```python
from build123d import *

# Parameters (mm, degrees)
SKETCH1_R           = 14.3
SKETCH1_R_2         = 12.7
BOSS_EXTRUDE1_DEPTH = 3.175
BOSS_EXTRUDE2_START = -0.635
SKETCH2_R           = 1.5875
BOSS_EXTRUDE2_DEPTH = 6.35
CIRPATTERN1_COUNT   = 2


with BuildPart() as part:
    # Sketch1 → Boss-Extrude1 (new body)
    with BuildSketch(Plane.XY):
        Circle(SKETCH1_R)
        Circle(SKETCH1_R_2, mode=Mode.SUBTRACT)
    extrude(amount=BOSS_EXTRUDE1_DEPTH)

    # Sketch2 → Boss-Extrude2 (add)
    with BuildSketch(Plane(origin=(14.3, 0, 0), x_dir=(0, 0, -1), z_dir=(1, 0, 0)).offset(BOSS_EXTRUDE2_START)):
        with Locations((-1.5875, 0)):
            Circle(SKETCH2_R)
    boss_extrude2 = extrude(amount=BOSS_EXTRUDE2_DEPTH)

    # CirPattern1: Boss-Extrude2 ×2 about axis
    cirpattern1_axis = Axis((0, 0, 3.175), (0, 0, -1))
    for i in range(1, CIRPATTERN1_COUNT):
        add(boss_extrude2.rotate(cirpattern1_axis, i * 360 / CIRPATTERN1_COUNT))


solid = part.part
```
Read the model definition and answer for the solid it produces. Units are mm, in the model's axes. A direction names the side the tool comes from. Give positions to 0.01 mm unless a question says otherwise; leave off trailing zeros. Write each loop counter-clockwise with the first axis right and the second up, starting at its lowest first coordinate (ties: lowest second). Pieces come first, ordered by that corner, then holes. Notation, with made-up numbers: (-36, -23.75) -> (10, -23.75) arc R10 ccw to (10, -13.75) -> close; hole circle Ø8 at (-11, -7). An arc over 180 degrees is marked (long way). Answer as a JSON object with one key per item and string values.
1) Straight lines are drawn through the part: probe 1 along Y at (x, z) = (0, 2.15); probe 2 along X at (y, z) = (-10, 2.05); probe 3 along X at (y, z) = (0.25, 0.35) (3 decimals). For each, find the intervals that lie inside material, in ascending order. Write a range as from..to.
Findings below:
{"probe 1": "y = -14.3..-12.7, 12.7..14.3", "probe 2": "x = -10.22..-7.83, 7.83..10.22", "probe 3": "x = -20.015..-12.698, 12.698..20.015"}
2) Section A-A on x = 0 is taken. Write down the section's boundary in (y, z) (3 decimals), then the cut area to 3 significant figures.
Findings below:
{"outline": "(-14.3, 0) -> (-12.7, 0) -> (-12.7, 3.175) -> (-14.3, 3.175) -> close; (12.7, 0) -> (14.3, 0) -> (14.3, 3.175) -> (12.7, 3.175) -> close", "area": "10.2 mm^2"}
3) For a pull along Y with two mould halves and no side action, classify faces 3 (the cylindrical face through (-2.75, -12.4, 1.57)), 4 (the cylindrical face through (-17.07, 0.61, 0.12)), 5 (the flat face through (20.015, 0, 2)) as pulls with the +Y half, pulls with the -Y half, needs draft (parallel to the pull), parting line crosses it, or undercut.
Findings below:
{"face 3": "undercut", "face 4": "parting line crosses it", "face 5": "needs draft"}
4) Flat-ended cylindrical pins translate along their axes: pin 1 Ø1 at (y, z) = (9.5, 1) entering from -X; pin 2 Ø1.5 at (x, z) = (-5.5, 1) entering from +Y; pin 3 Ø1.5 at (x, z) = (-1.5, 2.5) entering from -Y. Find the tip coordinate at first contact, or state that the pin passes through.
Findings below:
{"pin 1": "stops at x = -11.11", "pin 2": "stops at y = 13.49", "pin 3": "stops at y = -14.28"}
5) A tool of negligible diameter and unlimited length cuts with its end or side. For faces 1 (the cylindrical face through (17, 0, 0)), 2 (the flat face through (0, 13, 3.175)), from which of +Z, -Z, +X, -X, +Y, -Y can it reach the whole face along a straight path? Write none if from no direction.
Findings below:
{"face 1": "+X", "face 2": "+Z, +X, -X, +Y, -Y"}
6) Section C-C on y = 11.5 is taken. Write down the section's boundary in (x, z) (3 decimals), then the cut area to 3 significant figures.
Findings below:
{"outline": "(-8.499, 0) -> (-5.389, 0) -> (-5.389, 3.175) -> (-8.499, 3.175) -> close; (5.389, 0) -> (8.499, 0) -> (8.499, 3.175) -> (5.389, 3.175) -> close", "area": "19.8 mm^2"}
7) Section B-B on z = 1.5 is taken. Write down the section's boundary in (x, y) (3 decimals), then the cut area to 3 significant figures.
Findings below:
{"outline": "(-20.015, -1.585) -> (-14.212, -1.585) arc R14.3 ccw to (14.212, -1.585) -> (20.015, -1.585) -> (20.015, 1.585) -> (14.212, 1.585) arc R14.3 ccw to (-14.212, 1.585) -> (-20.015, 1.585) -> close; hole circle Ø25.4 at (0, 0)", "area": "172 mm^2"}
